Build history of the part. All positions in model axes, mm. A direction names the side the tool comes from. Round coordinates to 2 decimals unless told otherwise and drop trailing zeros. Write each loop counter-clockwise with the first axis right and the second up, starting at its lowest first coordinate (ties: lowest second). Pieces come first, ordered by that corner, then holes.
from build123d import *

# Parameters (mm, degrees)
F0_R     = 20
F1_DEPTH = 5
F2_R     = 15
F3_DEPTH = 5
F4_W     = 5
F4_H     = 19.364917
F5_DEPTH = 5


with BuildPart() as f1:
    # F0 (on Top) → F1 (new body)
    with BuildSketch(Plane.XY):
        Circle(F0_R)
    extrude(amount=F1_DEPTH)

    # F2 (on face) → F3 (join)
    with BuildSketch(Plane.XY.offset(5)):
        Circle(F2_R)
    extrude(amount=F3_DEPTH)

    # F4 (on face) → F5 (join)
    with BuildSketch(Plane.XY.offset(5)):
        with Locations((2.5, -9.682458)):
            Rectangle(F4_W, F4_H)
    extrude(amount=F5_DEPTH)


solid = f1.part
1) Slice it at B-B (y = -7). Write the cut outline in (x, z) (1 decimal).
Results:
outline: (-18.7, 0) - (18.7, 0) - (18.7, 5) - (13.3, 5) - (13.3, 10) - (-13.3, 10) - (-13.3, 5) - (-18.7, 5) - close
2) Wall check: L1, parallel to Z at x = 15, y = 7; L2, parallel to X at y = -0.5, z = 2.75; L3, parallel to X at y = 5.5, z = 4.5. Give the ranges that are in metal, low to high.
Results:
L1: z = 0 to 5
L2: x = -19.99 to 19.99
L3: x = -19.23 to 19.23
3) Slice it at A-A (x = 1). Write the cut outline in (y, z), plus the area to 3 significant figures.
Results:
outline: (-19.97, 0) - (19.97, 0) - (19.97, 5) - (14.97, 5) - (14.97, 10) - (-19.36, 10) - (-19.36, 5) - (-19.97, 5) - close
area: 371 mm2
4) Slice it at D-D (x = 17.5). Write the cut outline in (y, z), plus the area to 3 significant figures.
Results:
outline: (-9.68, 0) - (9.68, 0) - (9.68, 5) - (-9.68, 5) - close
area: 96.8 mm2
5) Which spindle directions (+Z, -Z, +X, -X, +Y, -Y) get a long thin tool onto all of the face, cutting with end or side? Do faces 1 (the cylindrical face through (-1.919, 14.877, 7.465)), 2 (the flat face through (5, -17, 7)), 3 (the flat face through (0, -17, 7)), 4 (the flat face through (2, -19.365, 7)). Say none if no direction does.
Results:
face 1: +Z
face 2: +Z, +X, -Y
face 3: +Z, -X, -Y
face 4: +Z, +X, -X, -Y
6) Slice it at C-C (z = 6). Write the cut outline in (x, y).
Results:
outline: (0, -19.36) - (5, -19.36) - (5, -14.14) arc R15 ccw (long way) to (0, -15) - close
7) Pin check, flat tips, straight feed: pin 1 Ø2.5 at (x, z) = (2.5, 7) entering from -Y; pin 2 Ø5 at (y, z) = (-13, 4.5) entering from +X; pin 3 Ø2.5 at (y, z) = (-16, 8.5) entering from +X. Stop position of each tip, or through.
Results:
pin 1: stops at y = -19.36
pin 2: stops at x = 17.02
pin 3: stops at x = 5
